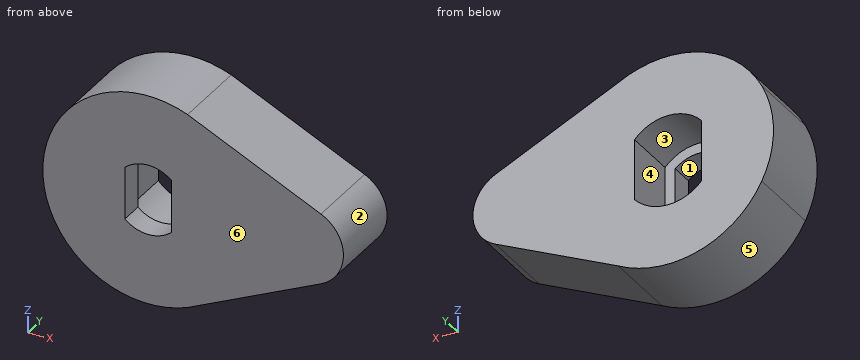
Autodesk Fusion 360 part; units mm, degrees
sketch "Sketch1" plane through (0, 0, 0) normal (0, 1, 0) x (1, 0, 0)
  arc A0 (-2, -13.1375) -> (2, -13.1375) centre (0, -11.25) ccw
  line L0 (-2, -13.1375) -> (-2, -9.3625)
  arc A1 (2, -9.3625) -> (-2, -9.3625) centre (0, -11.25) ccw
  line L1 (2, -9.3625) -> (2, -13.1375)
  line L2 (-2.15, -13.1962) -> (-2.15, -9.3038)
  arc A2 (2.15, -9.3038) -> (-2.15, -9.3038) centre (0, -11.25) ccw
  line L3 (2.15, -9.3038) -> (2.15, -13.1962)
  arc A3 (-2.15, -13.1962) -> (2.15, -13.1962) centre (0, -11.25) ccw
  arc A4 (-6, -14.3423) -> (6, -14.3423) centre (0, -11.25) ccw
  line L4 (6, -8.1577) -> (6, -14.3423)
  arc A5 (6, -8.1577) -> (-6, -8.1577) centre (0, -11.25) ccw
  line L5 (-6, -14.3423) -> (-6, -8.1577)
  circle A6 centre (10, -11.25) radius 2.5
  line L6 (2.5219, -17.5112) -> (11.06, -13.5142)
  line L7 (3.1933, -5.3031) -> (11.06, -8.9858)
  line L8 (1.5, -9.5729) -> (1.5, -12.9271)
  arc A7 (-1.5, -12.9271) -> (1.5, -12.9271) centre (0, -11.25) ccw
  line L9 (-1.5, -12.9271) -> (-1.5, -9.5729)
  arc A8 (1.5, -9.5729) -> (-1.5, -9.5729) centre (0, -11.25) ccw
  circle A9 centre (0, -11.25) radius 6.75
  dimension "d1" = 0.15
  dimension "d2" = -4
  dimension "d3" = 5
  dimension "d4" = 10
  dimension "d7" = 0.5
  dimension "d10" = 13.5
extrude "Extrude1" add sketch "Sketch1" along normal blind 5 contours A4 L4 A5 L5 L6 A9 | L5 A9 | A4 A5 A6 L6 L7 A9 | L4 A9 | A6
extrude "Extrude2" add sketch "Sketch1" along normal blind 1.5 contours A0 L0 A1 L1 | L2 A2 L3 A3
Can you work these out from the model? Positions are in its coordinate system, mm. Face numbers are marked on the shaded views. A direction names the side the tool comes from. Coordinates: 2 decimals unless noted, no trailing zeros. Order: outer loops, then holes, each group sorted by start corner. A loop starts at its lowest first (then second) coordinate and runs counter-clockwise, first axis right, second up.
1. If we section it at D-D (z = 16): Please give me the cut outline in (x, y), then the cut area to 3 significant figures.
2. For the marked faces 1, 2 and 3, which set-ups out of +Z, -Z, +X, -X, +Y, -Y let a thin tool reach every point of the face, with its end or its side?
3. If we section it at C-C (y = 0.3): Please give me the cut outline in (x, z).
4. Thinking about a two-plate mould opening in X: for the marked faces 4, 5 and 6, which applies, +X half, -X half, draft (parallel to the pull), parting line (faces both ways), or undercut?
5. I'm going to push flat-ended pins straight in: pin 1 (3 mm diameter, centred on y = 1.5, z = 6.5, fed in from +X); pin 2 (2 mm diameter, centred on y = 1, z = 13, fed in from +X); pin 3 (1.8 mm diameter, centred on y = 3.5, z = 10.5, fed in from -X); pin 4 (1.3 mm diameter, centred on x = 1, z = 11.5, fed in from +Y). Where does each tip first touch, or does it pass through?
6. I need wall thicknesses on line 1 (X direction, y = 0.95, z = 12.5); line 2 (X direction, y = 0.85, z = 12); line 3 (Z direction, x = -1, y = 1.35). Which ranges of each line are inside material? Lowest first, please.
7. If we section it at B-B (z = 11.5): Please give me the cut outline in (x, y).
8. If we section it at A-A (x = 0): Please give me the cut outline in (y, z), then the cut area to 3 significant figures.
Entries:
1. outline: (-4.8, 0) - (5.75, 0) - (5.75, 5) - (-4.8, 5) - close
1. area: 52.7 mm2
2. face 1: +Y, -Y
2. face 2: +X, +Y, -Y
2. face 3: +Y
3. outline: (2.52, 17.51) arc R6.75 ccw (long way) to (3.19, 5.3) - (11.06, 8.99) arc R2.5 ccw to (11.06, 13.51) - close; hole (-1.5, 9.57) arc R2.25 ccw to (1.5, 9.57) - (1.5, 12.93) arc R2.25 ccw to (-1.5, 12.93) - close
4. face 4: undercut
4. face 5: parting line
4. face 6: draft
5. pin 1: stops at x = 8.95
5. pin 2: stops at x = 12.38
5. pin 3: stops at x = -6.75
5. pin 4: stops at y = 1.5
6. line 1: x = -6.63 to -1.5, 1.5 to 12.17
6. line 2: x = -6.71 to -1.5, 1.5 to 12.38
6. line 3: z = 4.57 to 9.23, 13.27 to 17.93
7. outline: (-6.75, 0) - (-1.5, 0) - (-1.5, 1.5) - (-2.15, 1.5) - (-2.15, 5) - (-6.75, 5) - close; (1.5, 0) - (12.49, 0) - (12.49, 5) - (2.15, 5) - (2.15, 1.5) - (1.5, 1.5) - close
8. outline: (0, 4.5) - (5, 4.5) - (5, 8.35) - (1.5, 8.35) - (1.5, 9) - (0, 9) - close; (0, 13.5) - (1.5, 13.5) - (1.5, 14.15) - (5, 14.15) - (5, 18) - (0, 18) - close
8. area: 40.4 mm2
